```python
from build123d import *

# Parameters (mm, degrees)
SKETCH1_R           = 3.175
BOSS_EXTRUDE1_DEPTH = 1.5875
FILLET1_R           = 3.175


with BuildPart() as part:
    # Sketch1 → Boss-Extrude1 (new body)
    with BuildSketch(Plane.XY):
        with BuildLine():
            ThreePointArc((-12.7, 0), (-3.719743879, 3.719743879), (0, 12.7))
            Line((0, 12.7), (0, 38.1))
            ThreePointArc((0, 38.1), (-3.719743879, 47.080256121), (-12.7, 50.8))
            Line((-12.7, 50.8), (-41.275, 50.8))
            ThreePointArc((-41.275, 50.8), (-50.255256121, 47.080256121), (-53.975, 38.1))
            Line((-53.975, 38.1), (-53.975, 0))
            Line((-53.975, 0), (-53.975, -3.175))
            Line((-53.975, -3.175), (-25.4, -3.175))
            Line((-25.4, -3.175), (-25.4, 0))
            Line((-25.4, 0), (-12.7, 0))
        make_face()
        with Locations((-41.275, 9.525)):
            Circle(SKETCH1_R, mode=Mode.SUBTRACT)
        with Locations((-12.7, 9.525)):
            Circle(SKETCH1_R, mode=Mode.SUBTRACT)
        with Locations((-41.275, 38.1)):
            Circle(SKETCH1_R, mode=Mode.SUBTRACT)
        with Locations((-12.7, 38.1)):
            Circle(SKETCH1_R, mode=Mode.SUBTRACT)
    extrude(amount=BOSS_EXTRUDE1_DEPTH)

    # Fillet1
    fillet1_edges = [part.edges().sort_by_distance(p)[0] for p in [
        (-53.975, -3.175, 0.79375),
    ]]
    fillet(fillet1_edges, radius=FILLET1_R)


solid = part.part
```
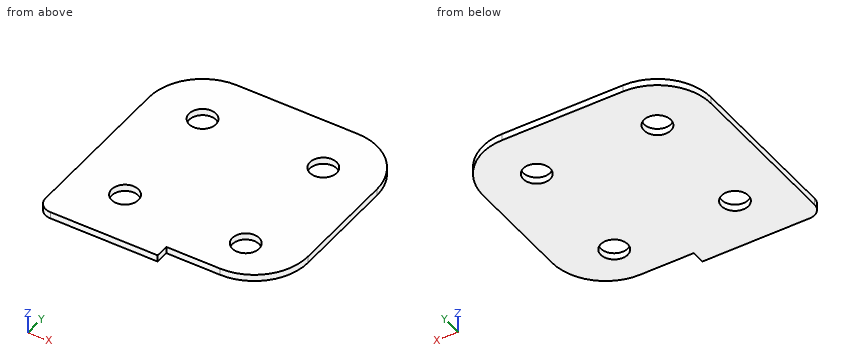
For this review, take the finished solid that the model builds, in its own axes (mm). Round coordinates to 2 decimals unless told otherwise and drop trailing zeros. Loops run counter-clockwise (first coordinate to the right, second up) from the corner with the lowest first, then second, coordinate; pieces in that order, holes last.
(1) Clearance check with flat-ended pins moving along their axes: P1, Ø0.8, axis at y = -1.5, z = 0.5, coming from the +X side; P2, Ø0.8, axis at x = -21, z = 1, coming from the -Y side; P3, Ø5.5, axis at x = -41.275, y = 9.525, coming from the -Z side. State where each tip first meets the part, or that it passes through.
Returned:
P1: stops at x = -25.4
P2: stops at y = 0
P3: passes through
(2) We need section C-C (x = -50). Give the boundary of the cut face in (y, z) (1 decimal), plus the area to 3 significant figures.
Returned:
outline: (-3.2, 0) - (47.3, 0) - (47.3, 1.6) - (-3.2, 1.6) - close
area: 80.2 mm2
(3) We need section B-B (z = 1.3). Give the boundary of the cut face in (x, y) (3 decimals).
Returned:
outline: (-53.975, 0) arc R3.175 ccw to (-50.8, -3.175) - (-25.4, -3.175) - (-25.4, 0) - (-12.7, 0) arc R12.7 ccw to (0, 12.7) - (0, 38.1) arc R12.7 ccw to (-12.7, 50.8) - (-41.275, 50.8) arc R12.7 ccw to (-53.975, 38.1) - close; hole circle Ø6.35 at (-41.275, 9.525); hole circle Ø6.35 at (-41.275, 38.1); hole circle Ø6.35 at (-12.7, 9.525); hole circle Ø6.35 at (-12.7, 38.1)
(4) We need section D-D (y = 4.5). Give the boundary of the cut face in (x, z) (1 decimal).
Returned:
outline: (-54, 0) - (-3, 0) - (-3, 1.6) - (-54, 1.6) - close
(5) We need section A-A (y = 40). Give the boundary of the cut face in (x, z).
Returned:
outline: (-53.83, 0) - (-43.82, 0) - (-43.82, 1.59) - (-53.83, 1.59) - close; (-38.73, 0) - (-15.24, 0) - (-15.24, 1.59) - (-38.73, 1.59) - close; (-10.16, 0) - (-0.14, 0) - (-0.14, 1.59) - (-10.16, 1.59) - close
(6) Wall thickness on line 1 along Y through (x, z) = (-12.7, 0.6) (3 decimals); line 2 along X through (y, z) = (11.5, 1.25) (3 decimals); line 3 along Y through (x, z) = (-12, 1.2): over which ranges is each line inside the solid? List them lowest first.
Returned:
line 1: y = 0 to 6.35, 12.7 to 34.925, 41.275 to 50.8
line 2: x = -53.975 to -43.761, -38.789 to -15.186, -10.214 to -0.057
line 3: y = 0.02 to 6.43, 12.62 to 35, 41.2 to 50.78
